Part model, mm, in its own coordinate system. A direction names the side the tool comes from. Give positions to 0.01 mm unless a question says otherwise; leave off trailing zeros. Write each loop counter-clockwise with the first axis right and the second up, starting at its lowest first coordinate (ties: lowest second). Pieces come first, ordered by that corner, then holes. Notation, with made-up numbers: M -19,-11 L 22,-11 A34 cw 22,19 Z; hole C -36.75,5 d8. An arc over 180 degrees is marked long. Use CSV: the item, a comma, the result in double quotes. Start each with the question number.
Item 1: Mould opens along Z. For faces 1 (the cylindrical face through (36.99, 2.28, -282.15)), 2 (the cylindrical face through (37.15, 2.28, -231.99)), 3 (the flat face through (-1, 4.5, -113)) say: released by +Z, released by -Z, zero draft, split by the parting line, or undercut.
Item 2: Cut at B-B (y = 3.55). Count the separate pieces of the cut face and the enclosed holes in it, then the cut area to 3 significant figures.
Item 3: Which spindle directions (+Z, -Z, +X, -X, +Y, -Y) get a long thin tool onto all of the face, cutting with end or side? Do faces 4 (the cylindrical face through (18.01, 2.28, -232.15)), 5 (the flat face through (60, 2, -240)). Say none if no direction does.
Item 4: Pin check, flat tips, straight feed: pin 1 (2.5 mm diameter, centred on x = -54, z = -162.55, fed in from -Y); pin 2 (5 mm diameter, centred on x = -67, z = -102.55, fed in from +Y). Stop position of each tip, or through.
Item 5: Cut at A-A (x = -11.5). List the corners of the cut face in (y, z), then the cut area to 3 significant figures.
Item 6: Drill centre lines: line 1 (X direction, y = 1.6, z = -60.5); line 2 (X direction, y = 3, z = -142); line 3 (Z direction, x = 26, y = 3.65). Where is each one in solid material? Low to high. Write a range as [from, to].
from build123d import *

# Parameters (mm, degrees)
EXTRUDE_1_DEPTH     = 4.5
SKETCH_3_R          = 1.75
CUT_EXTRUDE_2_DEPTH = 297.049404661
SKETCH_4_R          = 1.5
CUT_EXTRUDE_3_DEPTH = 297.049404661
FILLET_1_R          = 10
SKETCH_7_R          = 1.5
CUT_EXTRUDE_4_DEPTH = 297.049404661
SKETCH_8_R          = 1.5
CUT_EXTRUDE_5_DEPTH = 297.049404661
CUT_EXTRUDE_6_DEPTH = 297.049404661
SKETCH_10_R         = 5.5
CUT_EXTRUDE_7_DEPTH = 297.049404661
SKETCH_11_R         = 1.5
CUT_EXTRUDE_8_DEPTH = 297.049404661


with BuildPart() as part:
    # 草图1 → 凸台-拉伸1 (new body)
    with BuildSketch(Plane(origin=(0, 0, 0), x_dir=(1, 0, 0), z_dir=(0, 1, 0))):
        Polygon((-80, 0), (80, 0), (80, 210), (40, 270), (40, 285), (-80, 285), align=None)
    extrude(amount=EXTRUDE_1_DEPTH)

    # 草图3 → 切除-拉伸2 (cut, through all)
    with BuildSketch(Plane(origin=(0, 4.5, 0), x_dir=(1, 0, 0), z_dir=(0, 1, 0))):
        with Locations(Location((-2.95, 60.858418011, 0), (0, 0, 270))):
            Circle(SKETCH_3_R)
        with Locations(Location((21.25, 60.858418011, 0), (0, 0, 270))):
            Circle(SKETCH_3_R)
        with Locations(Location((21.25, 30.858418011, 0), (0, 0, 270))):
            Circle(SKETCH_3_R)
        with Locations(Location((-2.95, 30.858418011, 0), (0, 0, 270))):
            Circle(SKETCH_3_R)
    extrude(amount=-CUT_EXTRUDE_2_DEPTH, mode=Mode.SUBTRACT)

    # 草图4 → 切除-拉伸3 (cut, through all)
    with BuildSketch(Plane(origin=(0, 4.5, 0), x_dir=(1, 0, 0), z_dir=(0, 1, 0))):
        with Locations(Location((-60, 202.548224484, 0), (0, 0, 270))):
            Circle(SKETCH_4_R)
        with Locations(Location((-67, 162.548224484, 0), (0, 0, 270))):
            Circle(SKETCH_4_R)
        with Locations(Location((-54, 162.548224484, 0), (0, 0, 270))):
            Circle(SKETCH_4_R)
        with Locations(Location((-67, 102.548224484, 0), (0, 0, 270))):
            Circle(SKETCH_4_R)
        with Locations(Location((-54, 102.548224484, 0), (0, 0, 270))):
            Circle(SKETCH_4_R)
        with Locations(Location((-60, 62.548224484, 0), (0, 0, 270))):
            Circle(SKETCH_4_R)
        with Locations(Location((60, 62.548224484, 0), (0, 0, 270))):
            Circle(SKETCH_4_R)
        with Locations(Location((53, 102.548224484, 0), (0, 0, 270))):
            Circle(SKETCH_4_R)
        with Locations(Location((66, 102.548224484, 0), (0, 0, 270))):
            Circle(SKETCH_4_R)
        with Locations(Location((53, 162.548224484, 0), (0, 0, 270))):
            Circle(SKETCH_4_R)
        with Locations(Location((66, 162.548224484, 0), (0, 0, 270))):
            Circle(SKETCH_4_R)
        with Locations(Location((60, 202.548224484, 0), (0, 0, 270))):
            Circle(SKETCH_4_R)
    extrude(amount=-CUT_EXTRUDE_3_DEPTH, mode=Mode.SUBTRACT)

    # 圆角1
    fillet_1_edges = [part.edges().sort_by_distance(p)[0] for p in [
        (80, 2.25, 0),
        (-80, 2.25, 0),
        (-80, 2.25, -285),
        (40, 2.25, -285),
    ]]
    fillet(fillet_1_edges, radius=FILLET_1_R)

    # 草图7 → 切除-拉伸4 (cut, through all)
    with BuildSketch(Plane(origin=(0, 4.5, 0), x_dir=(1, 0, 0), z_dir=(0, 1, 0))):
        with Locations(Location((-62, 255, 0), (0, 0, 270))):
            Circle(SKETCH_7_R)
        with Locations(Location((-62, 225, 0), (0, 0, 270))):
            Circle(SKETCH_7_R)
    extrude(amount=-CUT_EXTRUDE_4_DEPTH, mode=Mode.SUBTRACT)

    # 草图8 → 切除-拉伸5 (cut, through all)
    with BuildSketch(Plane(origin=(0, 4.5, 0), x_dir=(1, 0, 0), z_dir=(0, 1, 0))):
        with Locations(Location((-0.5, 270, 0), (0, 0, 270))):
            Circle(SKETCH_8_R)
        with Locations(Location((-0.5, 255, 0), (0, 0, 270))):
            Circle(SKETCH_8_R)
        with Locations(Location((-0.5, 230, 0), (0, 0, 270))):
            Circle(SKETCH_8_R)
        with Locations(Location((-0.5, 200, 0), (0, 0, 270))):
            Circle(SKETCH_8_R)
    extrude(amount=-CUT_EXTRUDE_5_DEPTH, mode=Mode.SUBTRACT)

    # 草图9 → 切除-拉伸6 (cut, through all)
    with BuildSketch(Plane(origin=(0, 4.5, 0), x_dir=(1, 0, 0), z_dir=(0, 1, 0))):
        with BuildLine():
            Line((-30, 269), (-25, 269))
            ThreePointArc((-25, 269), (-17.928932188, 266.071067812), (-15, 259))
            Line((-15, 259), (-15, 199))
            ThreePointArc((-15, 199), (-17.928932188, 191.928932188), (-25, 189))
            Line((-25, 189), (-30, 189))
            ThreePointArc((-30, 189), (-37.071067812, 191.928932188), (-40, 199))
            Line((-40, 199), (-40, 259))
            ThreePointArc((-40, 259), (-37.071067812, 266.071067812), (-30, 269))
        make_face()
        with BuildLine():
            Line((25, 189), (30, 189))
            ThreePointArc((30, 189), (37.071067812, 191.928932188), (40, 199))
            Line((40, 199), (40, 225))
            ThreePointArc((40, 225), (37.071067812, 232.071067812), (30, 235))
            Line((30, 235), (25, 235))
            ThreePointArc((25, 235), (17.928932188, 232.071067812), (15, 225))
            Line((15, 225), (15, 199))
            ThreePointArc((15, 199), (17.928932188, 191.928932188), (25, 189))
        make_face()
        with BuildLine():
            Line((-35, 155), (35, 155))
            ThreePointArc((35, 155), (38.535533906, 153.535533906), (40, 150))
            Line((40, 150), (40, 140))
            ThreePointArc((40, 140), (38.535533906, 136.464466094), (35, 135))
            Line((35, 135), (-35, 135))
            ThreePointArc((-35, 135), (-38.535533906, 136.464466094), (-40, 140))
            Line((-40, 140), (-40, 150))
            ThreePointArc((-40, 150), (-38.535533906, 153.535533906), (-35, 155))
        make_face()
        with BuildLine():
            Line((-30, 112), (-15, 112))
            ThreePointArc((-15, 112), (-7.928932188, 109.071067812), (-5, 102))
            Line((-5, 102), (-5, 82))
            ThreePointArc((-5, 82), (-7.928932188, 74.928932188), (-15, 72))
            Line((-15, 72), (-30, 72))
            ThreePointArc((-30, 72), (-37.071067812, 74.928932188), (-40, 82))
            Line((-40, 82), (-40, 102))
            ThreePointArc((-40, 102), (-37.071067812, 109.071067812), (-30, 112))
        make_face()
        with BuildLine():
            Line((-54.5, 22.5), (-24.5, 22.5))
            ThreePointArc((-24.5, 22.5), (-20.964466094, 23.964466094), (-19.5, 27.5))
            Line((-19.5, 27.5), (-19.5, 37.5))
            ThreePointArc((-19.5, 37.5), (-20.964466094, 41.035533906), (-24.5, 42.5))
            Line((-24.5, 42.5), (-54.5, 42.5))
            ThreePointArc((-54.5, 42.5), (-58.035533906, 41.035533906), (-59.5, 37.5))
            Line((-59.5, 37.5), (-59.5, 27.5))
            ThreePointArc((-59.5, 27.5), (-58.035533906, 23.964466094), (-54.5, 22.5))
        make_face()
    extrude(amount=-CUT_EXTRUDE_6_DEPTH, mode=Mode.SUBTRACT)

    # 草图10 → 切除-拉伸7 (cut, through all)
    with BuildSketch(Plane(origin=(0, 4.5, 0), x_dir=(1, 0, 0), z_dir=(0, 1, 0))):
        with Locations(Location((-62, 240, 0), (0, 0, 270))):
            Circle(SKETCH_10_R)
    extrude(amount=-CUT_EXTRUDE_7_DEPTH, mode=Mode.SUBTRACT)

    # 草图11 → 切除-拉伸8 (cut, through all)
    with BuildSketch(Plane(origin=(0, 4.5, 0), x_dir=(1, 0, 0), z_dir=(0, 1, 0))):
        with Locations(Location((6, 93.669023571, 0), (0, 0, 270))):
            Circle(SKETCH_11_R)
        with Locations(Location((28, 93.669023571, 0), (0, 0, 270))):
            Circle(SKETCH_11_R)
        with Locations(Location((6, 71.669023571, 0), (0, 0, 270))):
            Circle(SKETCH_11_R)
        with Locations(Location((28, 71.669023571, 0), (0, 0, 270))):
            Circle(SKETCH_11_R)
    extrude(amount=-CUT_EXTRUDE_8_DEPTH, mode=Mode.SUBTRACT)


solid = part.part
Worked answers:
1,face 1,"released by -Z"
1,face 2,"undercut"
1,face 3,"zero draft"
2,separate pieces,"1"
2,enclosed holes,"32"
2,area,"36,800 mm^2"
3,face 4,"+Y, -Y"
3,face 5,"-Z, +X, +Y, -Y"
4,pin 1,"passes through"
4,pin 2,"stops at y = 4.5"
5,outline,"M 0,-285 L 4.5,-285 L 4.5,-155 L 0,-155 Z; M 0,-135 L 4.5,-135 L 4.5,-111.37 L 0,-111.37 Z; M 0,-72.63 L 4.5,-72.63 L 4.5,0 L 0,0 Z"
5,area,"1,020 mm^2"
6,line 1,"x = [-80, -4.66], [-1.24, 19.54], [22.96, 80]"
6,line 2,"x = [-80, -40], [40, 80]"
6,line 3,"z = [-285, -235], [-189, -155], [-135, 0]"
